Here's how the part is built. I have some questions about the finished solid (model axes, mm). Face numbers are marked on the shaded views. A direction names the side the tool comes from. Give positions to 0.01 mm unless a question says otherwise; leave off trailing zeros. Loops run counter-clockwise (first coordinate to the right, second up) from the corner with the lowest first, then second, coordinate; pieces in that order, holes last.
Q1. I'm going to push flat-ended pins straight in: P1, Ø2, axis at y = 33, z = 32, coming from the +X side; P2, Ø4, axis at x = 27.5, y = 28.5, coming from the +Z side. Where does each tip first touch, or does it pass through?
Q2. Suppose I cut it at A-A (x = 52.57). List the corners of the cut face in (y, z) for me (3 decimals).
Q3. Suppose I cut it at D-D (x = 29). List the corners of the cut face in (y, z) for me (3 decimals), and give its area (3 significant figures).
Q4. For the marked faces 1 and 2, which set-ups out of +Z, -Z, +X, -X, +Y, -Y let a thin tool reach every point of the face, with its end or its side?
Q5. Thinking about a two-plate mould opening in Y: for the marked faces 3, 4, 5 and 6, which applies, pulls with the +Y half, pulls with the -Y half, needs draft (parallel to the pull), parting line crosses it, or undercut?
Q6. I need wall thicknesses on probe 1 along Y at (x, z) = (5.43, 12.75) (3 decimals); probe 2 along Y at (x, z) = (29, 29.25) (3 decimals); probe 3 along Y at (x, z) = (52, 23). Which ranges of each line are inside material? Lowest first, please.
Q7. Suppose I cut it at C-C (z = 28). List the corners of the cut face in (x, y) for me (3 decimals), and give its area (3 significant figures).
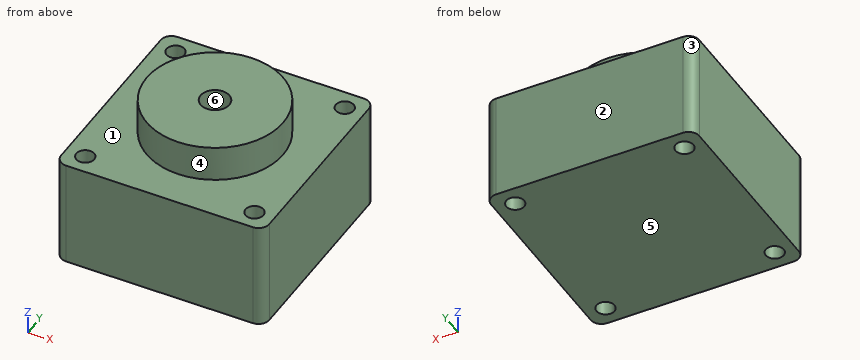
```python
from build123d import *

# Parameters (mm, degrees)
SKETCH_1_W          = 58
SKETCH_1_H          = 58
EXTRUDE_1_DEPTH     = 30
SKETCH_2_R          = 19.015
EXTRUDE_2_DEPTH     = 10
SKETCH_3_R          = 4.005
CUT_EXTRUDE_2_DEPTH = 25
SKETCH_4_R          = 2.505
CUT_EXTRUDE_3_DEPTH = 88.338422244
FILLET_1_R          = 3
FILLET_2_R          = 3
FILLET_3_R          = 3
FILLET_4_R          = 3


with BuildPart() as part:
    # 草图1 → 凸台-拉伸1 (new body)
    with BuildSketch(Plane.XY):
        with Locations((29, 29)):
            Rectangle(SKETCH_1_W, SKETCH_1_H)
    extrude(amount=EXTRUDE_1_DEPTH)

    # 草图2 → 凸台-拉伸2 (add)
    with BuildSketch(Plane.XY.offset(30)):
        with Locations((29, 29)):
            Circle(SKETCH_2_R)
    extrude(amount=EXTRUDE_2_DEPTH)

    # 草图3 → 切除-拉伸2 (cut)
    with BuildSketch(Plane.XY.offset(40)):
        with Locations((29, 29)):
            Circle(SKETCH_3_R)
    extrude(amount=-CUT_EXTRUDE_2_DEPTH, mode=Mode.SUBTRACT)

    # 草图4 → 切除-拉伸3 (cut, through all)
    with BuildSketch(Plane.XY.offset(30)):
        with Locations((52.57, 52.57)):
            Circle(SKETCH_4_R)
        with Locations((5.43, 52.57)):
            Circle(SKETCH_4_R)
        with Locations((5.43, 5.43)):
            Circle(SKETCH_4_R)
        with Locations((52.57, 5.43)):
            Circle(SKETCH_4_R)
    extrude(amount=-CUT_EXTRUDE_3_DEPTH, mode=Mode.SUBTRACT)

    # 圆角1
    fillet_1_edges = [part.edges().sort_by_distance(p)[0] for p in [
        (58, 58, 15),
    ]]
    fillet(fillet_1_edges, radius=FILLET_1_R)

    # 圆角2
    fillet_2_edges = [part.edges().sort_by_distance(p)[0] for p in [
        (58, 0, 15),
    ]]
    fillet(fillet_2_edges, radius=FILLET_2_R)

    # 圆角3
    fillet_3_edges = [part.edges().sort_by_distance(p)[0] for p in [
        (0, 58, 15),
    ]]
    fillet(fillet_3_edges, radius=FILLET_3_R)

    # 圆角4
    fillet_4_edges = [part.edges().sort_by_distance(p)[0] for p in [
        (0, 0, 15),
    ]]
    fillet(fillet_4_edges, radius=FILLET_4_R)


solid = part.part
```
Solutions:
1. P1: stops at x = 47.78
1. P2: stops at z = 15
2. outline: (0, 0) - (2.925, 0) - (2.925, 30) - (0, 30) - close; (7.935, 0) - (50.065, 0) - (50.065, 30) - (7.935, 30) - close; (55.075, 0) - (58, 0) - (58, 30) - (55.075, 30) - close
3. outline: (0, 0) - (58, 0) - (58, 30) - (48.015, 30) - (48.015, 40) - (33.005, 40) - (33.005, 15) - (24.995, 15) - (24.995, 40) - (9.985, 40) - (9.985, 30) - (0, 30) - close
3. area: 1,920 mm2
4. face 1: +Z
4. face 2: +Z, -Z, +X, -X, +Y
5. face 3: pulls with the +Y half
5. face 4: parting line crosses it
5. face 5: needs draft
5. face 6: undercut
6. probe 1: y = 0 to 2.925, 7.935 to 50.065, 55.075 to 58
6. probe 2: y = 0 to 24.995, 33.005 to 58
6. probe 3: y = 0 to 2.99, 7.87 to 50.13, 55.01 to 58
7. outline: (0, 3) arc R3 ccw to (3, 0) - (55, 0) arc R3 ccw to (58, 3) - (58, 55) arc R3 ccw to (55, 58) - (3, 58) arc R3 ccw to (0, 55) - close; hole circle Ø5.01 at (5.43, 5.43); hole circle Ø5.01 at (5.43, 52.57); hole circle Ø8.01 at (29, 29); hole circle Ø5.01 at (52.57, 5.43); hole circle Ø5.01 at (52.57, 52.57)
7. area: 3,230 mm2
